```python
from build123d import *

# Parameters (mm, degrees)
SKETCH1_W            = 40
SKETCH1_H            = 80
SKETCH1_W_2          = 27.4
SKETCH1_H_2          = 67.4
M8_CLEARANCE_HOLE1_D = 10


with BuildPart() as part:
    # Sweep1: sweep along a curve in space
    with BuildLine() as sweep1_path:
        add(Edge.make_bspline(
            [(0, 0, -350), (0, 0, 350)],
            knots=[0, 0, 1, 1], degree=1))
    # Sketch1 → Sweep1 (sweep)
    with BuildSketch(Plane.XY):
        Rectangle(SKETCH1_W, SKETCH1_H)
        Rectangle(SKETCH1_W_2, SKETCH1_H_2, mode=Mode.SUBTRACT)
    sweep(path=sweep1_path.line)

    # M8 Clearance Hole1 (through all)
    with Locations(Plane(origin=(20, 0, 0), x_dir=(0, 0, -1), z_dir=(1, 0, 0))):
        with Locations((26, 13), (26, -14)):
            m8_clearance_hole1 = Hole(M8_CLEARANCE_HOLE1_D / 2)

    # Mirror1: M8 Clearance Hole1 across plane
    add(m8_clearance_hole1.mirror(Plane.XY), mode=Mode.SUBTRACT)


solid = part.part
```
Input: part model. Units: mm. Frame: model coordinates. A direction names the side the tool comes from. Round coordinates to 2 decimals unless told otherwise and drop trailing zeros. Loops run counter-clockwise (first coordinate to the right, second up) from the corner with the lowest first, then second, coordinate; pieces in that order, holes last. Notation, with made-up numbers: (-12.75, -1.75) -> (30.25, -1.75) arc R32 ccw to (30.25, 37.25) -> close; hole circle Ø2 at (60, 82). An arc over 180 degrees is marked (long way). Use one line per item in the form item = value. Start each with the question number.
Item 1: Set-up query: faces 1 (the face through (0, 40, 5)), 2 (the face through (0, -33.7, 5)). Return all of +Z, -Z, +X, -X, +Y, -Y with unobstructed straight access to the full face (end or side cutting, diameter ignored); none if empty.
Item 2: Mould query, pull axis X, two halves, no side actions, for faces 3 (the face through (13.7, 0, 5)), 4 (the face through (-20, 1, 5)), 5 (the face through (-13.7, 0, 5)), 6 (the face through (-18, 1, 350)). Classes: pulls with the +X half, pulls with the -X half, needs draft (parallel to the pull), parting line crosses it, or undercut.
Item 3: Section query A-A on x = 2.5. Return the cut outline in (y, z), then the cut area to 3 significant figures.
Item 4: Material intervals for L1, parallel to Y at x = -17, z = 26; L2, parallel to Y at x = 0, z = -307; L3, parallel to X at y = -22.5, z = 160.5, sorted ascending. Write a range as from..to.
Item 5: Section query B-B on z = 113. Return the cut outline in (x, y).
Item 6: Contact query for flat-ended pins moving along their axis: pin 1 Ø6 at (y, z) = (13, -26) entering from +X; pin 2 Ø11.5 at (y, z) = (13, -26) entering from -X. Output: stop coordinate, or through.
Item 7: Section query C-C on y = 27. Return the cut outline in (x, z), then the cut area to 3 significant figures.
Ans:
q1.face_1 = +Z, -Z, +X, -X, +Y
q1.face_2 = +Z, -Z
q2.face_3 = undercut
q2.face_4 = pulls with the -X half
q2.face_5 = undercut
q2.face_6 = needs draft
q3.outline = (-40, -350) -> (-33.7, -350) -> (-33.7, 350) -> (-40, 350) -> close; (33.7, -350) -> (40, -350) -> (40, 350) -> (33.7, 350) -> close
q3.area = 8,820 mm^2
q4.L1 = -40..-19, -9..8, 18..40
q4.L2 = -40..-33.7, 33.7..40
q4.L3 = -20..-13.7, 13.7..20
q5.outline = (-20, -40) -> (20, -40) -> (20, 40) -> (-20, 40) -> close; hole (-13.7, -33.7) -> (13.7, -33.7) -> (13.7, 33.7) -> (-13.7, 33.7) -> close
q6.pin_1 = through
q6.pin_2 = -20
q7.outline = (-20, -350) -> (-13.7, -350) -> (-13.7, 350) -> (-20, 350) -> close; (13.7, -350) -> (20, -350) -> (20, 350) -> (13.7, 350) -> close
q7.area = 8,820 mm^2
